```python
from build123d import *

# Parameters (mm, degrees)
EXTRUDE_1_DEPTH     = 40
SKETCH_2_R          = 1.65
SKETCH_2_W          = 27
SKETCH_2_H          = 22
CUT_EXTRUDE_2_DEPTH = 10
SKETCH_3_R          = 2
CUT_EXTRUDE_3_DEPTH = 10
FILLET_1_R          = 3


with BuildPart() as part:
    # 草图1 → 凸台-拉伸1 (new body)
    with BuildSketch(Plane.XY):
        Polygon((0, 0), (30, 0), (30, -60), (27, -60), (27, -3), (0, -3), align=None)
    extrude(amount=EXTRUDE_1_DEPTH)

    # 草图2 → 切除-拉伸2 (cut)
    with BuildSketch(Plane(origin=(0, 0, 0), x_dir=(1, 0, 0), z_dir=(0, 1, 0))):
        with Locations((7.5, -4.5)):
            Circle(SKETCH_2_R)
        with Locations((19.5, -4.5)):
            Circle(SKETCH_2_R)
        with Locations((19.5, -35.5)):
            Circle(SKETCH_2_R)
        with Locations((7.5, -35.5)):
            Circle(SKETCH_2_R)
        with Locations((13.5, -20)):
            Rectangle(SKETCH_2_W, SKETCH_2_H)
    extrude(amount=-CUT_EXTRUDE_2_DEPTH, mode=Mode.SUBTRACT)

    # 草图3 → 切除-拉伸3 (cut)
    with BuildSketch(Plane(origin=(30, 0, 0), x_dir=(0, 0, -1), z_dir=(1, 0, 0))):
        with Locations((-25, -5)):
            Circle(SKETCH_3_R)
        with Locations((-15, -5)):
            Circle(SKETCH_3_R)
        with Locations((-15, -55)):
            Circle(SKETCH_3_R)
        with Locations((-25, -55)):
            Circle(SKETCH_3_R)
        Polygon((-20.75, -9.5), (-20.75, -2.75), (-19.25, -2.75), (-19.25, -9.5), (-9, -9.5), (-9, -50.5), (-19.25, -50.5), (-19.25, -57.25), (-20.75, -57.25), (-20.75, -50.5), (-31, -50.5), (-31, -9.5), align=None)
    extrude(amount=-CUT_EXTRUDE_3_DEPTH, mode=Mode.SUBTRACT)

    # 圆角1
    fillet_1_edges = [part.edges().sort_by_distance(p)[0] for p in [
        (27, -3, 35.5),
        (28.5, -60, 40),
        (27, -3, 4.5),
        (28.5, -60, 0),
        (28.5, -9.5, 19.25),
        (28.5, -50.5, 19.25),
        (28.5, -50.5, 20.75),
        (28.5, -9.5, 20.75),
    ]]
    fillet(fillet_1_edges, radius=FILLET_1_R)


solid = part.part
```
Design review of the part built by this model. Coordinates are the model's own, in mm. A direction names the side the tool comes from. Round coordinates to 2 decimals unless told otherwise and drop trailing zeros. Order: outer loops, then holes, each group sorted by start corner. A loop starts at its lowest first (then second) coordinate and runs counter-clockwise, first axis right, second up. Notation, with made-up numbers: (38.25, 18) - (57.25, 18) arc R19 ccw to (57.25, 54) - close; hole circle Ø6 at (15, 30.5). An arc over 180 degrees is marked (long way). One line per question, with ' | ' between items.
Item 1: Take a section at C-C, the plane y = -33. Write out the cut boundary in (x, z), then the cut area to 3 significant figures.
Checks:
outline: (27, 0) - (30, 0) - (30, 9) - (27, 9) - close; (27, 31) - (30, 31) - (30, 40) - (27, 40) - close | area: 54.0 mm²
Item 2: Draft analysis for pull direction Y (two halves, no side actions). For faces 5 (the face through (27.3, -22, 40)), 6 (the face through (29, -9.5, 27)), 7 (the face through (26.14, -3.9, 4.56)), state which applies: +Y half, -Y half, draft (parallel to the pull), parting line (faces both ways), or undercut.
Checks:
face 5: draft | face 6: undercut | face 7: -Y half
Item 3: Take a section at D-D, the plane x = 7.5. Write out the cut boundary in (y, z).
Checks:
outline: (-3, 0) - (0, 0) - (0, 2.85) - (-3, 2.85) - close; (-3, 6.15) - (0, 6.15) - (0, 9) - (-3, 9) - close; (-3, 31) - (0, 31) - (0, 33.85) - (-3, 33.85) - close; (-3, 37.15) - (0, 37.15) - (0, 40) - (-3, 40) - close
Item 4: Take a section at A-A, the plane x = 22.5. Write out the cut boundary in (y, z).
Checks:
outline: (-3, 0) - (0, 0) - (0, 9) - (-3, 9) - close; (-3, 31) - (0, 31) - (0, 40) - (-3, 40) - close
Item 5: Take a section at B-B, the plane z = 15. Write out the cut boundary in (x, y).
Checks:
outline: (27, -60) - (30, -60) - (30, -57) - (27, -57) - close; (27, -53) - (30, -53) - (30, -50.5) - (27, -50.5) - close; (27, -9.5) - (30, -9.5) - (30, -7) - (27, -7) - close; (27, -3) - (30, -3) - (30, 0) - (27, 0) - close
Item 6: For P1, Ø5, axis at x = 26, y = -10.5, coming from the +Z side; P2, Ø10, axis at x = 8.5, z = 13, coming from the -Y side; P3, Ø12, axis at y = -20, z = 4, coming from the -X side; P4, Ø3, axis at x = 19.5, z = 4.5, coming from the -Y side, all flat-tipped, find the tip position at first contact; note any pin that passes through.
Checks:
P1: z = 40 | P2: y = -3 | P3: x = 27 | P4: through
Item 7: Machinability: for faces 1 (the face through (29, -60, 20)), 2 (the face through (12, -3, 4)), 3 (the face through (13, -2, 31)), 4 (the face through (29, -30, 9)), which of the approach directions +Z, -Z, +X, -X, +Y, -Y give a long, thin tool a straight path to every point of the face, cutting with its end or side? Answer none if there is none.
Checks:
face 1: +Z, -Z, +X, -X, -Y | face 2: +Z, -Z, -X, -Y | face 3: -X, +Y, -Y | face 4: +X, -X
Item 8: Wall thickness on line 1 (X direction, y = -1.15, z = 4.5); line 2 (Z direction, x = 19.5, y = -2.15); line 3 (Y direction, x = 29.35, z = 15): over which ranges is each line inside the solid? List them lowest first. Write a range as [from, to].
Checks:
line 1: [0, 5.85], [9.15, 17.85], [21.15, 30] | line 2: [0, 2.85], [6.15, 9], [31, 33.85], [37.15, 40] | line 3: [-60, -57], [-53, -50.5], [-9.5, -7], [-3, 0]
